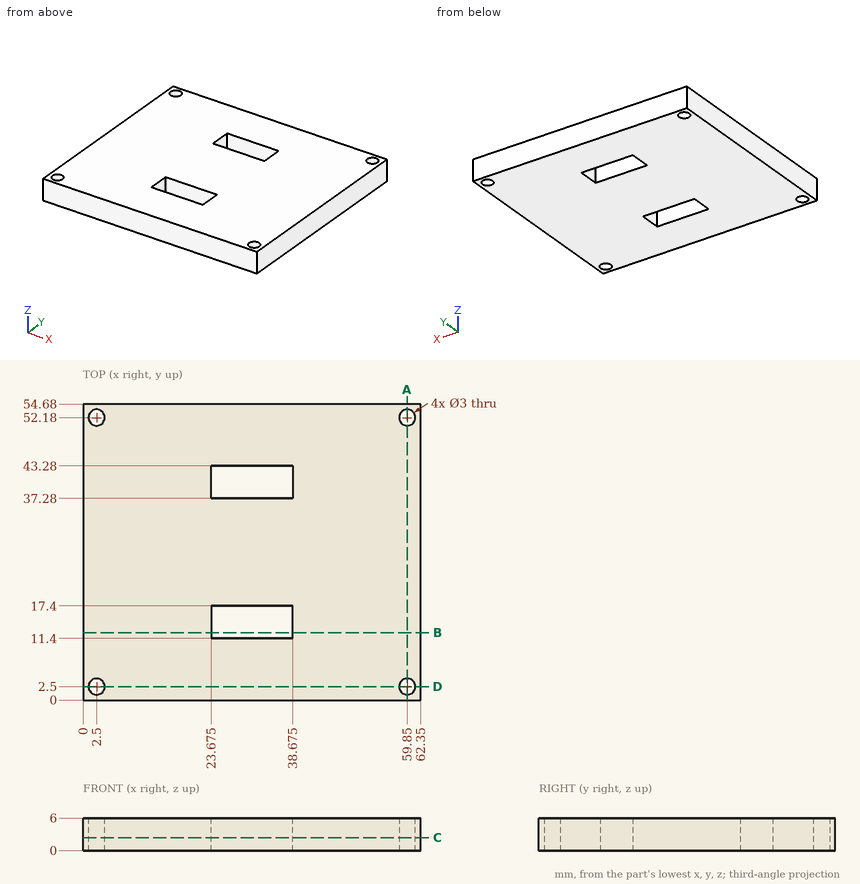
Could you check a few things on this drawing? It's one solid part, dimensions in mm from its lowest x, y, z. Coordinates: 2 decimals unless noted, no trailing zeros. Write each loop counter-clockwise with the first axis right and the second up, starting at its lowest first coordinate (ties: lowest second). Pieces come first, ordered by that corner, then holes. Notation, with made-up numbers: M 82,-1 L 103,-1 A4 cw 103,5 Z; hole C -28.75,5 d1. An arc over 180 degrees is marked long. Answer as CSV lines item,"result". Start each with the question number.
Q1. Suppose I cut it at B-B, the plane y = 12.5. List the corners of the cut face in (x, z) for me (3 decimals).
Q2. Suppose I cut it at A-A, the plane x = 59.85. List the corners of the cut face in (y, z) for me.
Q3. Suppose I cut it at D-D, the plane y = 2.5. List the corners of the cut face in (x, z) for me, then the cut area to 3 significant figures.
Q4. I need wall thicknesses on probe 1 along Y at (x, z) = (59.85, 4.4); probe 2 along Y at (x, z) = (29, 4.8); probe 3 along X at (y, z) = (12.5, 0.7) (3 decimals). Which ranges of each line are inside material? Lowest first, please. Write a range as [from, to].
Q5. Suppose I cut it at C-C, the plane z = 2.4. List the corners of the cut face in (x, y) for me (3 decimals), then the cut area to 3 significant figures.
Entries:
1,outline,"M 0,0 L 23.675,0 L 23.675,6 L 0,6 Z; M 38.675,0 L 62.35,0 L 62.35,6 L 38.675,6 Z"
2,outline,"M 0,0 L 1,0 L 1,6 L 0,6 Z; M 4,0 L 50.68,0 L 50.68,6 L 4,6 Z; M 53.68,0 L 54.68,0 L 54.68,6 L 53.68,6 Z"
3,outline,"M 0,0 L 1,0 L 1,6 L 0,6 Z; M 4,0 L 58.35,0 L 58.35,6 L 4,6 Z; M 61.35,0 L 62.35,0 L 62.35,6 L 61.35,6 Z"
3,area,"338 mm²"
4,probe 1,"y = [0, 1], [4, 50.68], [53.68, 54.68]"
4,probe 2,"y = [0, 11.4], [17.4, 37.28], [43.28, 54.68]"
4,probe 3,"x = [0, 23.675], [38.675, 62.35]"
5,outline,"M 0,0 L 62.35,0 L 62.35,54.68 L 0,54.68 Z; hole C 2.5,2.5 d3; hole C 2.5,52.18 d3; hole M 23.675,11.4 L 38.675,11.4 L 38.675,17.4 L 23.675,17.4 Z; hole M 23.675,37.28 L 38.675,37.28 L 38.675,43.28 L 23.675,43.28 Z; hole C 59.85,2.5 d3; hole C 59.85,52.18 d3"
5,area,"3,200 mm²"
